from build123d import *

# Parameters (mm, degrees)
F0_W      = 26
F0_H      = 88
F1_DEPTH  = 30
F2_DEPTH  = 30
F3_R      = 5
F4_R      = 10.1474815612
F5_DEPTH  = 5
F6_R      = 7.5
F7_DEPTH  = 15
F8_R      = 6.4108279614
F9_DEPTH  = 15
F10_W     = 12.5
F10_H     = 80
F11_DEPTH = 1
F12_W     = 16
F12_H     = 52
F13_DEPTH = 5
F14_W     = 3
F14_H     = 44.2491837641
F15_DEPTH = 16
F16_W     = 0.5
F16_H     = 3.3036185751
F17_DEPTH = 16


with BuildPart() as f1:
    # F0 (on Front) → F1 (new body)
    with BuildSketch(Plane.XZ):
        Rectangle(F0_W, F0_H)
    extrude(amount=F1_DEPTH)

    # F2 (add): a face of the model
    f2_faces = [f1.faces().sort_by_distance(p)[0] for p in [
        (0, 0, 0),
    ]]
    extrude(f2_faces, amount=F2_DEPTH)

    # F3
    f3_edges = [f1.edges().sort_by_distance(p)[0] for p in [
        (13, 30, 0),
        (-13, 30, 0),
        (-13, -30, 0),
        (13, -30, 0),
    ]]
    fillet(f3_edges, radius=F3_R)

    # F4 (on face) → F5 (join)
    with BuildSketch(Plane.XY.offset(44)):
        with Locations((0, -16.4110772312)):
            Circle(F4_R)
    extrude(amount=F5_DEPTH)

    # F6 (on face) → F7 (join)
    with BuildSketch(Plane.XY.offset(49)):
        with Locations((0, -16.4110772312)):
            Circle(F6_R)
    extrude(amount=F7_DEPTH)

    # F8 (on face) → F9 (cut)
    with BuildSketch(Plane.XY.offset(64)):
        with Locations((0, -16.4110772312)):
            Circle(F8_R)
    extrude(amount=-F9_DEPTH, mode=Mode.SUBTRACT)

    # F10 (on face) → F11 (cut)
    with BuildSketch(Plane.YZ.offset(13)):
        with Locations((-13.4554863907, 0)):
            Rectangle(F10_W, F10_H)
    extrude(amount=-F11_DEPTH, mode=Mode.SUBTRACT)

    # F12 (on face) → F13 (join)
    with BuildSketch(Plane(origin=(-13, 0, 0), x_dir=(0, -1, 0), z_dir=(-1, 0, 0))):
        with Locations((0, -4)):
            Rectangle(F12_W, F12_H)
    extrude(amount=F13_DEPTH)

    # F14 (on face) → F15 (cut)
    with BuildSketch(Plane.XZ.offset(8)):
        with Locations((-14.5, -4.5717895428)):
            Rectangle(F14_W, F14_H)
    extrude(amount=-F15_DEPTH, mode=Mode.SUBTRACT)

    # F16 (on face) → F17 (cut)
    with BuildSketch(Plane.XZ.offset(8)):
        with Locations((-13.25, -28.3481907124)):
            Rectangle(F16_W, F16_H)
    extrude(amount=-F17_DEPTH, mode=Mode.SUBTRACT)


solid = f1.part
Can you work these out from the model? Positions are in its coordinate system, mm. A direction names the side the tool comes from. Coordinates: 2 decimals unless noted, no trailing zeros. Order: outer loops, then holes, each group sorted by start corner. A loop starts at its lowest first (then second) coordinate and runs counter-clockwise, first axis right, second up. Notation, with made-up numbers: (27.25, 19) - (31.25, 19) arc R28 ccw to (31.25, 44) - close; hole circle Ø6 at (21, -30). An arc over 180 degrees is marked (long way). Answer as a JSON object with one key per item and string values. Group by question number.
Q1. Imagine slicing it at B-B (x = 0). Please give me the cut outline in (y, z), and give its area (3 significant figures).
Q2. I need wall thicknesses on line 1 (X direction, y = -3.5, z = 3); line 2 (Y direction, x = 0, z = 53.25); line 3 (X direction, y = -15, z = 30). Which ranges of each line are inside material? Lowest first, please. Write a range as from..to.
Q3. On a 3-axis mill with a long thin cutter (end or side, diameter ignored), from which of +Z, -Z, +X, -X, +Y, -Y can I reach the whole of each face in a straight line? I mean faces 4 (the face through (-16, 0, -30)), 5 (the face through (-15, 0, -26.696)), 6 (the face through (-17, -8, -4)), 7 (the face through (-15, 0, 22)). Say none if no direction works.
Q4. Imagine slicing it at D-D (y = 20). Please give me the cut outline in (x, z), and give its area (3 significant figures).
Q5. We'd pull the mould along X, two halves only. Please class faces 1 (the face through (0, -30, 1)), 2 (the face through (12, 28, 1)), 3 (the face through (-15, 0, 17.553)): +X half, -X half, draft (parallel to the pull), parting line (faces both ways), or undercut.
Q6. Imagine slicing it at C-C (z = 29.5). Please give me the cut outline in (x, y).
Q7. Will these pins go through, and if not, where does the flat tip stop? P1, Ø5, axis at x = -5.5, y = 0, coming from the +Z side; P2, Ø1.5, axis at x = -15.5, y = 2.5, coming from the +Z side; P3, Ø5, axis at x = -15, z = -11, coming from the -Y side; P4, Ø2.5, axis at x = -14, y = 0.5, coming from the -Z side.
Q8. Imagine slicing it at A-A (z = -12.5). Please give me the cut outline in (x, y), and give its area (3 significant figures).
Determined:
{
 "1": {"outline": "(-30, -44) - (30, -44) - (30, 44) - (-6.26, 44) - (-6.26, 49) - (-8.91, 49) - (-8.91, 64) - (-10, 64) - (-10, 49) - (-22.82, 49) - (-22.82, 64) - (-23.91, 64) - (-23.91, 49) - (-26.56, 49) - (-26.56, 44) - (-30, 44) - close", "area": "5,410 mm2"},
 "2": {"line 1": "x = -18..-16, -13..13", "line 2": "y = -23.91..-22.82, -10..-8.91", "line 3": "x = -13..12"},
 "3": {"face 4": "-Z, -X, +Y, -Y", "face 5": "+Y, -Y", "face 6": "+Z, -Z, -X, -Y", "face 7": "+Z, -X, +Y, -Y"},
 "4": {"outline": "(-13, -44) - (13, -44) - (13, 44) - (-13, 44) - close", "area": "2,290 mm2"},
 "5": {"face 1": "draft", "face 2": "+X half", "face 3": "undercut"},
 "6": {"outline": "(-13, -25) arc R5 ccw to (-8, -30) - (8, -30) arc R5 ccw to (13, -25) - (13, -19.71) - (12, -19.71) - (12, -7.21) - (13, -7.21) - (13, 25) arc R5 ccw to (8, 30) - (-8, 30) arc R5 ccw to (-13, 25) - close"},
 "7": {"P1": "stops at z = 44", "P2": "stops at z = 22", "P3": "stops at y = -27.18", "P4": "stops at z = -44"},
 "8": {"outline": "(-18, -8) - (-16, -8) - (-16, 8) - (-18, 8) - close; (-13, -25) arc R5 ccw to (-8, -30) - (8, -30) arc R5 ccw to (13, -25) - (13, -19.71) - (12, -19.71) - (12, -7.21) - (13, -7.21) - (13, 25) arc R5 ccw to (8, 30) - (-8, 30) arc R5 ccw to (-13, 25) - close", "area": "1,560 mm2"}
}
